Solid Edge part; units mm, degrees
sketch "Sketch1" plane through (23.4359, 29.9999, -20) normal (0, 0, -1) x (-0.024896, -0.99969, 0)
  arc A0 (-14.815, 12.5282) -> (-12.9235, 14.1753) centre (-0.103, -2.457) cw
  line L0 (-29.4072, 14.1753) -> (-12.9235, 14.1753)
  line L1 (-29.4072, 24.1753) -> (-29.4072, 14.1753)
  line L2 (-29.4072, 24.1753) -> (30.5741, 22.6818)
  line L3 (30.5741, 22.6818) -> (30.3252, 12.6849)
  line L4 (30.3252, 12.6849) -> (14.0129, 13.091)
  line L5 (-15.7497, -16.4635) -> (-15.1524, -15.5764)
  line L6 (-14.815, 12.5282) -> (-13.4055, 12.5282)
  arc A1 (14.0129, 13.091) -> (-15.7497, -16.4635) centre (-0.103, -2.4571) cw
  arc A2 (-13.4055, 12.5282) -> (-15.1524, -15.5765) centre (-0.8135, -2.3611) cw
extrude "Protrusion1" add sketch "Sketch1" against normal blind 20
sketch "Sketch2" plane through (5.0002, -0.0001, -10) normal (0, -1, 0) x (1, 0, 0)
  line L0 (-5.0001, 10.0001) -> (-5.0001, -9.9998)
  line L1 (-5.0001, -9.9998) -> (-0.1985, 10.0001)
  line L2 (-0.1985, 10.0001) -> (-5.0001, 10.0001)
extrude "ExtrudedCutout_2" cut sketch "Sketch2" against normal blind 84.595
Here's how the part is built. I have some questions about the finished solid (model axes, mm). Coordinates: 2 decimals unless noted, no trailing zeros. Order: outer loops, then holes, each group sorted by start corner. A loop starts at its lowest first (then second) coordinate and runs counter-clockwise, first axis right, second up. Notation, with made-up numbers: M 43.5,-12.75 L 80.5,-12.75 A29 cw 80.5,21.25 Z; hole C 21,88 d11. An arc over 180 degrees is marked long. Answer as a JSON object with one key per item and string values. Group by question number.
(1) I need wall thicknesses on probe 1 along Y at (x, z) = (26.5, -18.25); probe 2 along X at (y, z) = (25.5, -10.25); probe 3 along Y at (x, z) = (9.5, -14.5). Which ranges of each line are inside material? Lowest first, please.
(2) For pin 1 (6 mm diameter, centred on x = 41, z = -12.5, fed in from +Y); pin 2 (5 mm diameter, centred on x = 41.5, z = -5.5, fed in from -Y); pin 3 (12 mm diameter, centred on y = 16, z = -7, fed in from -X); pin 4 (23.5 mm diameter, centred on x = 25.82, y = 30.75, fed in from -Z), each with a flat end and sliding along its axis, tell me the tip position at first contact or that it passes through.
(3) If we mould it in two halves opening along X, with no side actions, what happens to faces 1 (the face through (2.367, 29.58, -10.14)), 2 (the face through (27.178, 11.302, -10.14)), 3 (the face through (6, 30, -20))? For each: released by +X, released by -X, zero draft, split by the parting line, or undercut.
(4) Suppose I cut it at C-C, the plane y = 13. State how many separate pieces and enclosed holes the cut face has, then the cut area to 3 significant figures.
(5) Suppose I cut it at B-B, the plane z = -13.75. Please give me the cut outline in (x, y), then the cut area to 3 significant figures.
Values found:
{
 "1": {"probe 1": "y = 9.05 to 11.27", "probe 2": "x = 2.34 to 7.04, 44.6 to 46.4", "probe 3": "y = 0 to 20.08, 41.43 to 59.76"},
 "2": {"pin 1": "stops at y = 45.33", "pin 2": "stops at y = 13.63", "pin 3": "stops at x = 1.68", "pin 4": "passes through"},
 "3": {"face 1": "released by -X", "face 2": "undercut", "face 3": "zero draft"},
 "4": {"separate pieces": "3", "enclosed holes": "0", "area": "320 mm^2"},
 "5": {"outline": "M 1.5,0 L 10,0 L 10,16.32 A21 ccw long 40.29,45.33 L 39.38,44.76 A19.5 cw long 11.25,43.71 L 11.28,45.12 A21 ccw 9.59,43.27 L 10,59.75 L 1.5,59.96 Z", "area": "573 mm^2"}
}
